```python
from build123d import *

# Parameters (mm, degrees)
F0_W            = 4
F0_H            = 10
F1_ANGLE_BACK   = 110
F1_ANGLE        = 220
F2_ANGLE_START  = 60
F2_ANGLE        = 30
F3_ANGLE_START  = 60
F3_ANGLE        = 30
F4_ANGLE_BACK   = 15
F4_ANGLE        = 30
F5_R            = 4
F6_DEPTH        = 10
F7_R            = 5
F8_SIZE         = 5
F9_W            = 10
F9_H            = 1
F10_ANGLE_START = 7
F10_ANGLE       = 13
F11_ANGLE_START = 7
F11_ANGLE       = 13
F12_ANGLE_START = 82
F12_ANGLE       = 13
F13_ANGLE_START = 82
F13_ANGLE       = 13
F14_ANGLE_START = 55
F14_ANGLE       = 13
F15_ANGLE_START = 55
F15_ANGLE       = 13


with BuildPart() as f1:
    # F0 (on Front) → F1 (revolve)
    with BuildSketch(Plane.XZ, mode=Mode.PRIVATE) as f1_sk:
        with Locations((26, 10)):
            Rectangle(F0_W, F0_H)
    revolve(f1_sk.sketch.rotate(Axis((0, 0, 10), (0, 0, 1)), -F1_ANGLE_BACK), axis=Axis((0, 0, 10), (0, 0, 1)), revolution_arc=F1_ANGLE)

    # F0 (on Front) → F2 (revolve)
    with BuildSketch(Plane.XZ, mode=Mode.PRIVATE) as f2_sk:
        Polygon((24, 21.5), (24, 15), (28, 15), (28, 24.5), (13, 24.5), (13, 21.5), align=None)
        Polygon((28, 5), (24, 5), (24, 0), (17, 0), (17, -1), (20, -2), (28, -2), align=None)
    revolve(f2_sk.sketch.rotate(Axis((0, 0, 10), (0, 0, -1)), F2_ANGLE_START), axis=Axis((0, 0, 10), (0, 0, -1)), revolution_arc=F2_ANGLE)

    # F0 (on Front) → F3 (revolve)
    with BuildSketch(Plane.XZ, mode=Mode.PRIVATE) as f3_sk:
        Polygon((24, 21.5), (24, 15), (28, 15), (28, 24.5), (13, 24.5), (13, 21.5), align=None)
        Polygon((28, 5), (24, 5), (24, 0), (17, 0), (17, -1), (20, -2), (28, -2), align=None)
    revolve(f3_sk.sketch.rotate(Axis((0, 0, 10), (0, 0, 1)), F3_ANGLE_START), axis=Axis((0, 0, 10), (0, 0, 1)), revolution_arc=F3_ANGLE)

    # F0 (on Front) → F4 (revolve)
    with BuildSketch(Plane.XZ, mode=Mode.PRIVATE) as f4_sk:
        Polygon((24, 21.5), (24, 15), (28, 15), (28, 24.5), (13, 24.5), (13, 21.5), align=None)
        Polygon((28, 5), (24, 5), (24, 0), (17, 0), (17, -1), (20, -2), (28, -2), align=None)
    revolve(f4_sk.sketch.rotate(Axis((0, 0, 10), (0, 0, 1)), -F4_ANGLE_BACK), axis=Axis((0, 0, 10), (0, 0, 1)), revolution_arc=F4_ANGLE)

    # F5 (on face) → F6 (join, through all)
    with BuildSketch(Plane.XY.offset(15)):
        with Locations((-8.2084834398, 22.5526228989)):
            Circle(F5_R)
        with Locations((-8.2084834398, -22.5526228989)):
            Circle(F5_R)
    extrude(amount=-F6_DEPTH)

    # F7
    f7_edges = [f1.edges().sort_by_distance(p)[0] for p in [
        (24, 0, 21.5),
        (6.211657, 23.18222, 21.5),
        (6.211657, -23.18222, 21.5),
        (6.211657, -23.18222, 0),
        (6.211657, 23.18222, 0),
        (24, 0, 0),
    ]]
    fillet(f7_edges, radius=F7_R)

    # F8
    f8_edges = [f1.edges().sort_by_distance(p)[0] for p in [
        (7.246933, 27.045923, 24.5),
        (28, 0, 24.5),
        (7.246933, -27.045923, 24.5),
        (7.246933, -27.045923, -2),
        (7.246933, 27.045923, -2),
        (28, 0, -2),
    ]]
    chamfer(f8_edges, length=F8_SIZE)

    # F9 (on Front) → F10 (revolve, cut)
    with BuildSketch(Plane.XZ, mode=Mode.PRIVATE) as f10_sk:
        with Locations((27, 15.5)):
            Rectangle(F9_W, F9_H)
        with Locations((27, 4.5)):
            Rectangle(F9_W, F9_H)
    revolve(f10_sk.sketch.rotate(Axis((0, 0, 10), (0, 0, -1)), F10_ANGLE_START), axis=Axis((0, 0, 10), (0, 0, -1)), revolution_arc=F10_ANGLE, mode=Mode.SUBTRACT)

    # F9 (on Front) → F11 (revolve, cut)
    with BuildSketch(Plane.XZ, mode=Mode.PRIVATE) as f11_sk:
        with Locations((27, 15.5)):
            Rectangle(F9_W, F9_H)
        with Locations((27, 4.5)):
            Rectangle(F9_W, F9_H)
    revolve(f11_sk.sketch.rotate(Axis((0, 0, 10), (0, 0, 1)), F11_ANGLE_START), axis=Axis((0, 0, 10), (0, 0, 1)), revolution_arc=F11_ANGLE, mode=Mode.SUBTRACT)

    # F9 (on Front) → F12 (revolve, cut)
    with BuildSketch(Plane.XZ, mode=Mode.PRIVATE) as f12_sk:
        with Locations((27, 15.5)):
            Rectangle(F9_W, F9_H)
        with Locations((27, 4.5)):
            Rectangle(F9_W, F9_H)
    revolve(f12_sk.sketch.rotate(Axis((0, 0, 10), (0, 0, 1)), F12_ANGLE_START), axis=Axis((0, 0, 10), (0, 0, 1)), revolution_arc=F12_ANGLE, mode=Mode.SUBTRACT)

    # F9 (on Front) → F13 (revolve, cut)
    with BuildSketch(Plane.XZ, mode=Mode.PRIVATE) as f13_sk:
        with Locations((27, 15.5)):
            Rectangle(F9_W, F9_H)
        with Locations((27, 4.5)):
            Rectangle(F9_W, F9_H)
    revolve(f13_sk.sketch.rotate(Axis((0, 0, 10), (0, 0, -1)), F13_ANGLE_START), axis=Axis((0, 0, 10), (0, 0, -1)), revolution_arc=F13_ANGLE, mode=Mode.SUBTRACT)

    # F9 (on Front) → F14 (revolve, cut)
    with BuildSketch(Plane.XZ, mode=Mode.PRIVATE) as f14_sk:
        with Locations((27, 15.5)):
            Rectangle(F9_W, F9_H)
        with Locations((27, 4.5)):
            Rectangle(F9_W, F9_H)
    revolve(f14_sk.sketch.rotate(Axis((0, 0, 10), (0, 0, -1)), F14_ANGLE_START), axis=Axis((0, 0, 10), (0, 0, -1)), revolution_arc=F14_ANGLE, mode=Mode.SUBTRACT)

    # F9 (on Front) → F15 (revolve, cut)
    with BuildSketch(Plane.XZ, mode=Mode.PRIVATE) as f15_sk:
        with Locations((27, 15.5)):
            Rectangle(F9_W, F9_H)
        with Locations((27, 4.5)):
            Rectangle(F9_W, F9_H)
    revolve(f15_sk.sketch.rotate(Axis((0, 0, 10), (0, 0, 1)), F15_ANGLE_START), axis=Axis((0, 0, 10), (0, 0, 1)), revolution_arc=F15_ANGLE, mode=Mode.SUBTRACT)


solid = f1.part
```
Could you check a few things on this model? Use its own coordinates, in mm. A direction names the side the tool comes from. Coordinates: 2 decimals unless noted, no trailing zeros. Write each loop counter-clockwise with the first axis right and the second up, starting at its lowest first coordinate (ties: lowest second). Pieces come first, ordered by that corner, then holes. Notation, with made-up numbers: (53, -4.75) -> (101, -4.75) arc R23 ccw to (101, 10.25) -> close; hole circle Ø4 at (-1.5, 63). An arc over 180 degrees is marked (long way). Write item = value, one per line. Start each with the question number.
(1) Which directions (+Z, -Z, +X, -X, +Y, -Y) give clear straight access to the entire face, cutting with the end or side of a thin tool? Please do faces 1 (the face through (0, 24, 1)), 2 (the face through (3.411, 12.545, 22.979)), 3 (the face through (11, 23, 16)).
(2) Will these pins go through, and if not, where does the flat tip stop? pin 1 (1.9 mm diameter, centred on x = 1.5, y = 26.5, fed in from +Z); pin 2 (2 mm diameter, centred on x = 6.5, z = 18, fed in from -Y); pin 3 (8 mm diameter, centred on x = -1, y = 21, fed in from -Z); pin 4 (1.3 mm diameter, centred on x = 26.5, y = 4, fed in from +Z).
(3) I want a section at C-C (z = 22.5). Please give me the cut outline in (x, y).
(4) We'd pull the mould along Y, two halves only. Please class faces 4 (the face through (-5, -24, 5)), 5 (the face through (6.681, -24.573, 0.465)), 6 (the face through (18.2, -0.1, -1.4)): released by +Y, released by -Y, zero draft, split by the parting line, or undercut.
(5) I want a section at A-A (z = 17.25). Please give me the cut outline in (x, y).
(6) I need wall thicknesses on line 1 (Y direction, x = 0, z = 14); line 2 (Y direction, x = -10, z = 10.5); line 3 (Y direction, x = 25, z = 9.5). Which ranges of each line are inside material? Lowest first, please. Write a range as [from, to].
(7) I want a section at D-D (y = -21.5). Give the number of separate pieces and of enclosed holes in the cut face, plus the area to 3 significant figures.
(8) I want a section at B-B (y = 0). Please give me the cut outline in (x, z), plus the area to 3 significant figures.
Result set:
q1.face_1 = -Z, -X, +Y, -Y
q1.face_2 = +Z, -Z, -X
q1.face_3 = +X
q2.pin_1 = 21.91
q2.pin_2 = -27.45
q2.pin_3 = -2
q2.pin_4 = 21.35
q3.outline = (0, -25) arc R25 ccw to (12.5, -21.65) -> (6.5, -11.26) arc R13 cw to (0, -13) -> close; (0, 13) arc R13 cw to (6.5, 11.26) -> (12.5, 21.65) arc R25 ccw to (0, 25) -> close; (12.56, -3.36) -> (24.15, -6.47) arc R25 ccw to (24.15, 6.47) -> (12.56, 3.36) arc R13 cw to start
q4.face_4 = zero draft
q4.face_5 = released by -Y
q4.face_6 = undercut
q5.outline = (0, -28) arc R28 ccw to (14, -24.25) -> (11.97, -20.74) arc R23.94 cw to (0, -23.94) -> close; (0, 23.94) arc R23.94 cw to (11.97, 20.74) -> (14, 24.25) arc R28 ccw to (0, 28) -> close; (23.13, -6.2) -> (27.05, -7.25) arc R28 ccw to (27.05, 7.25) -> (23.13, 6.2) arc R23.94 cw to start
q6.line_1 = [-28, -24], [24, 28]
q6.line_2 = [-26.13, -18.98], [18.98, 26.13]
q6.line_3 = [-12.61, 12.61]
q7.separate_pieces = 4
q7.enclosed_holes = 0
q7.area = 253 mm2
q8.outline = (13, 21.5) -> (19, 21.5) arc R5 cw to (24, 16.5) -> (24, 5) arc R5 cw to (19, 0) -> (17, 0) -> (17, -1) -> (20, -2) -> (23, -2) -> (28, 3) -> (28, 19.5) -> (23, 24.5) -> (13, 24.5) -> close
q8.area = 137 mm2
